Could you check a few things on this drawing? It's one solid part, dimensions in mm from its lowest x, y, z. Give positions to 0.01 mm unless a question says otherwise; leave off trailing zeros. Loops run counter-clockwise (first coordinate to the right, second up) from the corner with the lowest first, then second, coordinate; pieces in that order, holes last. Notation, with made-up numbers: (63.5, 87.5) -> (86.5, 87.5) arc R28 cw to (86.5, 115.5) -> close; hole circle Ø3 at (2, 7). An arc over 180 degrees is marked (long way). One line per question, with ' | ' between items.
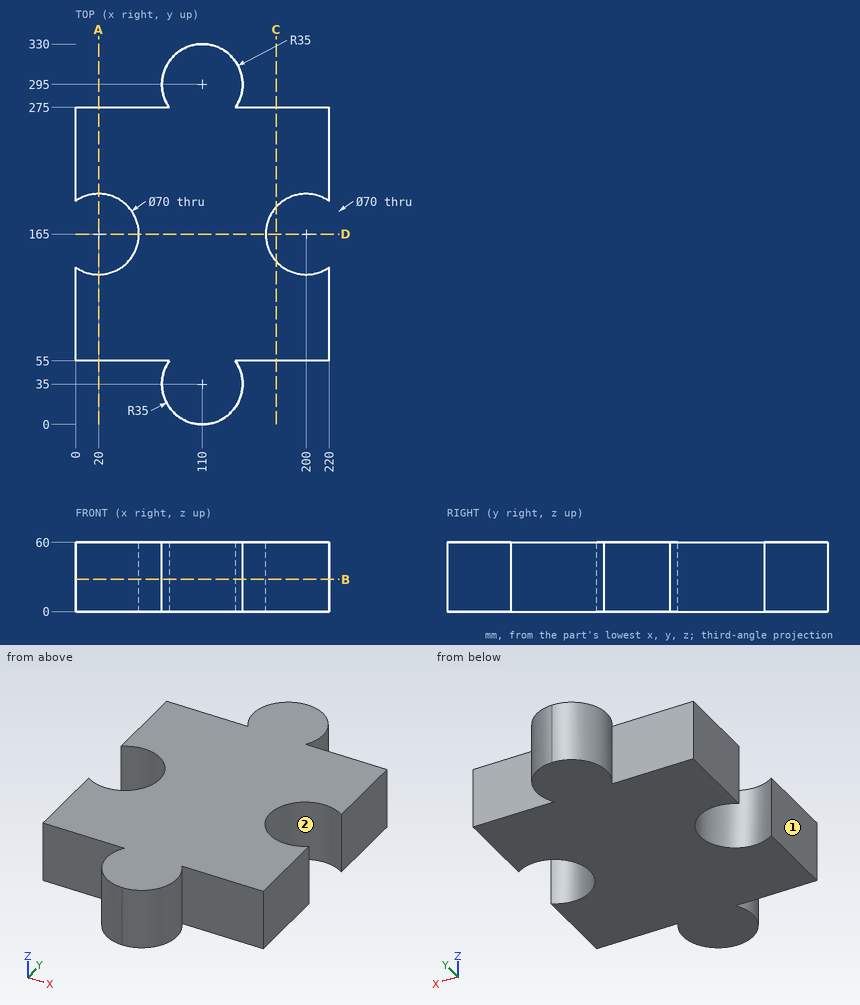
Q1. If we mould it in two halves opening along Y, with no side actions, what happens to the marked faces 1 and 2? For each: pulls with the +Y half, pulls with the -Y half, needs draft (parallel to the pull), parting line crosses it, or undercut.
Entries:
face 1: needs draft | face 2: undercut
Q2. For pin 1 Ø18 at (x, z) = (188, 39) entering from -Y; pin 2 Ø8 at (y, z) = (164.5, 10.5) entering from +X, each with a flat end and sliding along its axis, tell me the tip position at first contact or that it passes through.
Entries:
pin 1: y = 55 | pin 2: x = 165.29
Q3. If we section it at A-A (x = 20): Write out the boundary of the cut face in (y, z), plus the area to 3 significant figures.
Entries:
outline: (55, 0) -> (130, 0) -> (130, 60) -> (55, 60) -> close; (200, 0) -> (275, 0) -> (275, 60) -> (200, 60) -> close | area: 9,000 mm²
Q4. If I drill on probe 1 along Y at (x, z) = (20, 27); probe 2 along Y at (x, z) = (176.5, 35); probe 3 along Y at (x, z) = (72, 21), over which ranges is the centre line in solid material (lowest first)? Write a range as from..to.
Entries:
probe 1: 55..130, 200..275 | probe 2: 55..139.06, 190.94..275 | probe 3: 55..275
Q5. If we section it at B-B (z = 28): Write out the boundary of the cut face in (x, y), plus the area to 3 significant figures.
Entries:
outline: (0, 55) -> (81.28, 55) arc R35 ccw (long way) to (138.72, 55) -> (220, 55) -> (220, 136.28) arc R35 cw (long way) to (220, 193.72) -> (220, 275) -> (138.72, 275) arc R35 ccw (long way) to (81.28, 275) -> (0, 275) -> (0, 193.72) arc R35 cw (long way) to (0, 136.28) -> close | area: 48,400 mm²
Q6. If we section it at C-C (x = 174): Write out the boundary of the cut face in (y, z).
Entries:
outline: (55, 0) -> (141.57, 0) -> (141.57, 60) -> (55, 60) -> close; (188.43, 0) -> (275, 0) -> (275, 60) -> (188.43, 60) -> close
Q7. If we section it at D-D (y = 165): Write out the boundary of the cut face in (x, z), plus the area to 3 significant figures.
Entries:
outline: (55, 0) -> (165, 0) -> (165, 60) -> (55, 60) -> close | area: 6,600 mm²
